```python
from build123d import *


with BuildPart() as part:
    # Sketch1 → Revolve1 (revolve)
    with BuildSketch(Plane.XY, mode=Mode.PRIVATE) as revolve1_sk:
        with BuildLine():
            Line((5, 0.95), (5, 1.851651123))
            Line((5, 1.851651123), (4.85, 2))
            Line((4.85, 2), (2.648348877, 2))
            Line((2.648348877, 2), (2.5, 1.851651123))
            Line((2.5, 1.851651123), (2.5, 0.453458929))
            ThreePointArc((2.5, 0.453458929), (2.675, 0), (2.5, -0.453458929))
            Line((2.5, -0.453458929), (2.5, -1.85))
            Line((2.5, -1.85), (2.648348877, -2))
            Line((2.648348877, -2), (4.85, -2))
            Line((4.85, -2), (5, -1.85))
            Line((5, -1.85), (5, -0.95))
            Line((5, -0.95), (4.85, -0.8))
            Line((4.85, -0.8), (4.2, -0.8))
            Line((4.2, -0.8), (4.2, -0.675))
            ThreePointArc((4.2, -0.675), (4.875, 0), (4.2, 0.675))
            Line((4.2, 0.675), (4.2, 0.8))
            Line((4.2, 0.8), (4.85, 0.8))
            Line((4.85, 0.8), (5, 0.95))
        make_face()
    revolve(revolve1_sk.sketch.rotate(Axis((0, -7.575237451, 0), (0, 1, 0)), 90), axis=Axis((0, -7.575237451, 0), (0, 1, 0)))


solid = part.part
```
Geometry: final body of the model. Coordinates: model frame, mm. A direction names the side the tool comes from. Coordinates: 2 decimals unless noted, no trailing zeros. Order: outer loops, then holes, each group sorted by start corner. A loop starts at its lowest first (then second) coordinate and runs counter-clockwise, first axis right, second up. Notation, with made-up numbers: (56.5, 85) - (65.5, 85) arc R16 cw to (65.5, 89) - close; hole circle Ø9 at (57.5, 61.25). An arc over 180 degrees is marked (long way). Write each question's results on one line, items separated by ' | '.
(1) First-contact query: pin 1 Ø3 at (x, z) = (1, -0.5) entering from -Y; pin 2 Ø1.5 at (x, z) = (-0.5, -0.5) entering from -Y; pin 3 Ø1.5 at (y, z) = (0, -1) entering from +X; pin 4 Ø2 at (y, z) = (0, 3) entering from -X. Flat tips, straight axial feed; report the tip coordinate or a pass-through.
Values found:
pin 1: stops at y = -1.97 | pin 2: passes through | pin 3: stops at x = 4.87 | pin 4: stops at x = -4.45
(2) Line query: line 1 (X direction, y = 1.15, z = 0); line 2 (Y direction, x = 4.75, z = 0.25); line 3 (Y direction, x = 4.75, z = -0.75). Output: solid intervals per line, ascending. Write a range as [from, to].
Values found:
line 1: x = [-5, -2.5], [2.5, 5] | line 2: y = [-2, -0.8], [-0.38, 0.38], [0.8, 2] | line 3: y = [-2, -0.8], [-0.29, 0.29], [0.8, 2]
(3) Section query A-A, the plane y = 1.6. Return the cut outline in (x, z), plus the area to 3 significant figures.
Values found:
outline: circle Ø10 at (0, 0); hole circle Ø5 at (0, 0) | area: 58.9 mm²
(4) Mould query, pull axis Y, two halves, no side actions, for faces 1 (the face through (2, 2, -2)), 2 (the face through (-2, 0.8, -4)), 3 (the face through (-0.22, 1.407, 4.995)), 4 (the face through (2, -2, 2)). Classes: +Y half, -Y half, draft (parallel to the pull), parting line (faces both ways), or undercut.
Values found:
face 1: +Y half | face 2: undercut | face 3: draft | face 4: -Y half
(5) Set-up query: faces 5 (the face through (-2, -0.8, 4)), 6 (the face through (-0.22, -1.394, 4.995)). Return all of +Z, -Z, +X, -X, +Y, -Y with unobstructed straight access to the full face (end or side cutting, diameter ignored); none if empty.
Values found:
face 5: none | face 6: +Y, -Y
